```python
from build123d import *

# Parameters (mm, degrees)
SKETCH1_R               = 34.384
SKETCH1_R_2             = 24.384
BOSS_EXTRUDE1_DEPTH     = 35
BOSS_EXTRUDE2_START     = -34
SKETCH1_3_R             = 34.384
BOSS_EXTRUDE2_DEPTH     = 34
CHAMFER1_SIZE           = 2
FILLET2_R               = 5
CUT_EXTRUDE1_DEPTH      = 3.571875
CUT_EXTRUDE1_DEPTH_BACK = 3.571875
F_10_0MM_DOWEL_HOLE1_D  = 10


with BuildPart() as part:
    # Sketch1 → Boss-Extrude1 (new body)
    with BuildSketch(Plane(origin=(0, 0, 0), x_dir=(1, 0, 0), z_dir=(0, 1, 0))):
        with Locations(Location((0, 0, 0), (0, 0, 270))):
            Circle(SKETCH1_R)
        with Locations(Location((0, 0, 0), (0, 0, 270))):
            Circle(SKETCH1_R_2, mode=Mode.SUBTRACT)
    extrude(amount=BOSS_EXTRUDE1_DEPTH)

    # Sketch1_3 → Boss-Extrude2 (add)
    with BuildSketch(Plane(origin=(0, 0, 0), x_dir=(1, 0, 0), z_dir=(0, 1, 0)).offset(BOSS_EXTRUDE2_START)):
        with Locations(Location((0, 0, 0), (0, 0, 270))):
            Circle(SKETCH1_3_R)
    extrude(amount=BOSS_EXTRUDE2_DEPTH)

    # Chamfer1
    chamfer1_edges = [part.edges().sort_by_distance(p)[0] for p in [
        (0, 35, -24.384),
    ]]
    chamfer(chamfer1_edges, length=CHAMFER1_SIZE)

    # Fillet2
    fillet2_edges = [part.edges().sort_by_distance(p)[0] for p in [
        (0, 35, -26.384),
        (0, 35, -34.384),
    ]]
    fillet(fillet2_edges, radius=FILLET2_R)

    # Sketch10 → Cut-Extrude1 (cut, two sides: drawn at the far end of the back side and taken through both)
    with BuildSketch(Plane(origin=(0, -22, 0), x_dir=(-1, 0, 0), z_dir=(0, -1, 0)).offset(-CUT_EXTRUDE1_DEPTH_BACK)):
        Polygon((7.332348419, 0), (3.666174209, 6.35), (-3.666174209, 6.35), (-7.332348419, 0), (-3.666174209, -6.35), (3.666174209, -6.35), align=None)
    extrude(amount=CUT_EXTRUDE1_DEPTH + CUT_EXTRUDE1_DEPTH_BACK, mode=Mode.SUBTRACT)

    # 10.0mm Dowel Hole1 (through all)
    with Locations(Plane(origin=(0, -34, 0), x_dir=(-1, 0, 0), z_dir=(0, -1, 0))):
        with Locations((0, 0)):
            Hole(F_10_0MM_DOWEL_HOLE1_D / 2)


solid = part.part
```
Verification items for the finished model (mm, model axes). A direction names the side the tool comes from. Round coordinates to 2 decimals unless told otherwise and drop trailing zeros. Order: outer loops, then holes, each group sorted by start corner. A loop starts at its lowest first (then second) coordinate and runs counter-clockwise, first axis right, second up. Notation, with made-up numbers: (12.25, -28) - (50.25, -28) arc R38 ccw to (50.25, 11) - close; hole circle Ø9 at (19, 39.5). An arc over 180 degrees is marked (long way). Use CSV: the item, a comma, the result in double quotes.
(1) Gauge pin test, flat ends, axial feed: pin 1 Ø10 at (x, z) = (-1.5, 2) entering from -Y; pin 2 Ø1 at (y, z) = (-9.5, -6.5) entering from +X; pin 3 Ø10 at (x, z) = (-0.5, 2.5) entering from +Y; pin 4 Ø1 at (x, y) = (17, -12.5) entering from +Z. Record the tip position at first contact, or that the pin passes through.
Entries:
pin 1,"y = -34"
pin 2,"x = 33.86"
pin 3,"y = 0"
pin 4,"z = 30.17"
(2) Mould release check, pull along X, two halves, no side actions. Record for faces 1 (the face through (10.328, -2.448, 32.796)), 2 (the face through (-5.525, -21.95, -3.131)), 3 (the face through (0, -34, 7)): released by +X, released by -X, zero draft, split by the parting line, or undercut.
Entries:
face 1,"split by the parting line"
face 2,"undercut"
face 3,"zero draft"
(3) Section check C-C on y = 4. Record the boundary of the cut face in (x, z).
Entries:
outline,"circle Ø68.77 at (0, 0); hole circle Ø48.77 at (0, 0)"
(4) Thickness scan on probe 1 along X at (y, z) = (19.5, 0); probe 2 along X at (y, z) = (16.5, -12.5); probe 3 along Z at (x, y) = (13.5, 27). Record the ranges inside material, lowest first. Write a range as from..to.
Entries:
probe 1,"-34.38..-24.38, 24.38..34.38"
probe 2,"-32.03..-20.94, 20.94..32.03"
probe 3,"-31.62..-20.31, 20.31..31.62"
(5) Section check A-A on y = -23. Record the boundary of the cut face in (x, z), and give its area (3 significant figures).
Entries:
outline,"circle Ø68.77 at (0, 0); hole (-7.33, 0) - (-3.67, -6.35) - (3.67, -6.35) - (7.33, 0) - (3.67, 6.35) - (-3.67, 6.35) - close"
area,"3,570 mm^2"
(6) Section check B-B on x = 0. Record the boundary of the cut face in (y, z).
Entries:
outline,"(-34, -34.38) - (30, -34.38) arc R5 ccw to (35, -29.38) - (35, -28.46) arc R5 ccw to (33.54, -24.92) - (33, -24.38) - (0, -24.38) - (0, -5) - (-18.43, -5) - (-18.43, -6.35) - (-25.57, -6.35) - (-25.57, -5) - (-34, -5) - close; (-34, 5) - (-25.57, 5) - (-25.57, 6.35) - (-18.43, 6.35) - (-18.43, 5) - (0, 5) - (0, 24.38) - (33, 24.38) - (33.54, 24.92) arc R5 ccw to (35, 28.46) - (35, 29.38) arc R5 ccw to (30, 34.38) - (-34, 34.38) - close"
(7) Access from +Z, -Z, +X, -X, +Y, -Y to the whole of each face (thin tool, end or side, straight path). Record for faces 4 (the face through (6, 0, 0)), 5 (the face through (0, -22, -6.35)), 6 (the face through (-1.08, -29.73, 4.88)).
Entries:
face 4,"+Y"
face 5,"none"
face 6,"+Y, -Y"
